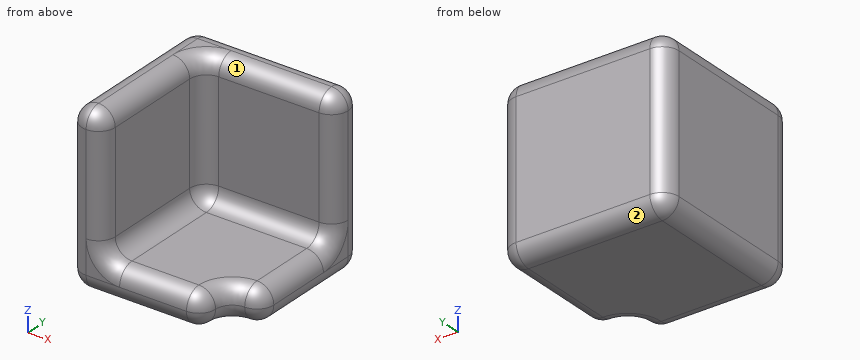
from build123d import *

# Parameters (mm, degrees)
F0_W     = 63.5
F0_H     = 63.5
F1_DEPTH = 63.5
F2_W     = 50.8
F2_H     = 50.8
F3_DEPTH = 50.8
F4_W     = 12.7
F4_H     = 12.7
F5_DEPTH = 12.7
F6_R     = 6.34999


# Not quite as in the source:
# - a fillet or chamfer is up to 0.001 mm smaller than in the source, because OpenCascade refuses the exact size


with BuildPart() as f1:
    # F0 (on Front) → F1 (new body)
    with BuildSketch(Plane.XZ):
        with Locations((31.75, -31.75)):
            Rectangle(F0_W, F0_H)
    extrude(amount=F1_DEPTH)

    # F2 (on face) → F3 (cut)
    with BuildSketch(Plane.XY):
        with Locations((38.1, -38.1)):
            Rectangle(F2_W, F2_H)
    extrude(amount=-F3_DEPTH, mode=Mode.SUBTRACT)

    # F4 (on face) → F5 (cut)
    with BuildSketch(Plane.XY.offset(-50.8)):
        with Locations((57.15, -57.15)):
            Rectangle(F4_W, F4_H)
    extrude(amount=-F5_DEPTH, mode=Mode.SUBTRACT)

    # F6 (radius 6.35 in the source; OpenCascade refuses exactly that, so slightly less here)
    f6_edges = [f1.edges().sort_by_distance(p)[0] for p in [
        (31.75, 0, 0),
        (0, -31.75, 0),
        (6.35, -63.5, 0),
        (12.7, -38.1, 0),
        (38.1, -12.7, 0),
        (63.5, -6.35, 0),
        (63.5, -50.8, -57.15),
        (50.8, -50.8, -57.15),
        (57.15, -50.8, -50.8),
        (57.15, -50.8, -63.5),
        (38.1, -12.7, -50.8),
        (63.5, -31.75, -50.8),
        (50.8, -57.15, -50.8),
        (31.75, -63.5, -50.8),
        (12.7, -38.1, -50.8),
        (63.5, 0, -31.75),
        (63.5, -12.7, -25.4),
        (63.5, -25.4, -63.5),
        (12.7, -63.5, -25.4),
        (50.8, -63.5, -57.15),
        (25.4, -63.5, -63.5),
        (0, -63.5, -31.75),
        (50.8, -57.15, -63.5),
        (31.75, 0, -63.5),
        (0, -31.75, -63.5),
        (12.7, -12.7, -25.4),
        (0, 0, -31.75),
    ]]
    fillet(f6_edges, radius=F6_R)


solid = f1.part
Design review of the part built by this model. Coordinates are the model's own, in mm. Face numbers are marked on the shaded views. A direction names the side the tool comes from. Round coordinates to 2 decimals unless told otherwise and drop trailing zeros. Return JSON: item names as keys, results as strings. Group by question number.
Item 1: Machinability: for the marked faces 1 and 2, which of the approach directions +Z, -Z, +X, -X, +Y, -Y give a long, thin tool a straight path to every point of the face, cutting with its end or side? Answer none if there is none.
Item 2: Insertion check: P1, Ø8, axis at x = 49.5, y = -56.5, coming from the +Z side; P2, Ø5, axis at x = 57, y = -21, coming from the +Z side; P3, Ø1, axis at x = 56.5, z = -34, coming from the -Y side. Each pin has a flat end and moves straight along its axis. Give the tip position at first contact, or say it passes through.
Item 3: For probe 1 along X at (y, z) = (-24, -27.5); probe 2 along Z at (x, y) = (23, -49); probe 3 along Y at (x, z) = (42, -32), list the stretches that pass through material, from the lowest coordinate up. Write a range as [from, to].
Model answer:
{
 "1": {"face 1": "+Z, +X, -Y", "face 2": "-Z, +X, -X, +Y"},
 "2": {"P1": "stops at z = -50.88", "P2": "stops at z = -50.78", "P3": "stops at y = -12.7"},
 "3": {"probe 1": "x = [0, 12.7]", "probe 2": "z = [-63.5, -50.8]", "probe 3": "y = [-12.7, 0]"}
}
